Here's how the part is built. I have some questions about the finished solid (model axes, mm). A direction names the side the tool comes from. Coordinates: 2 decimals unless noted, no trailing zeros. Write each loop counter-clockwise with the first axis right and the second up, starting at its lowest first coordinate (ties: lowest second). Pieces come first, ordered by that corner, then holes. Notation, with made-up numbers: M 66,76.25 L 89,76.25 A10 cw 89,85.25 Z; hole C 63.5,-3.5 d5. An arc over 180 degrees is marked long. Write each question's results on one line, items separated by ' | '. Start each with the question number.
from build123d import *

# Parameters (mm, degrees)
F0_W     = 103.023604
F0_H     = 61.1
F0_R     = 2
F1_DEPTH = 2
F2_R     = 5
F3_SIZE  = 0.4


with BuildPart() as f1:
    # F0 (on Top) → F1 (new body)
    with BuildSketch(Plane.XY):
        Rectangle(F0_W, F0_H)
        with Locations((-47.05, -24.27)):
            Circle(F0_R, mode=Mode.SUBTRACT)
        with BuildLine():
            ThreePointArc((49.05, -24.27), (47.05, -26.27), (45.05, -24.27))
            ThreePointArc((45.05, -24.27), (47.05, -22.27), (49.05, -24.27))
        make_face(mode=Mode.SUBTRACT)
        with Locations((-47.05, 24.27)):
            Circle(F0_R, mode=Mode.SUBTRACT)
        Polygon((43.8, -28.2), (-43.8, -28.2), (-43.8, 28.2), (43.8, 28.2), (43.8, -24.27), align=None, mode=Mode.SUBTRACT)
        with Locations((47.05, 24.27)):
            Circle(F0_R, mode=Mode.SUBTRACT)
    extrude(amount=F1_DEPTH)

    # F2
    f2_edges = [f1.edges().sort_by_distance(p)[0] for p in [
        (51.511802, -30.55, 1),
        (51.511802, 30.55, 1),
        (-51.511802, -30.55, 1),
        (-51.511802, 30.55, 1),
    ]]
    fillet(f2_edges, radius=F2_R)

    # F3
    f3_edges = [f1.edges().sort_by_distance(p)[0] for p in [
        (45.05, -24.27, 2),
        (45.05, 24.27, 2),
        (-49.05, 24.27, 2),
        (-49.05, -24.27, 2),
    ]]
    chamfer(f3_edges, length=F3_SIZE)


solid = f1.part
1) I want a section at C-C, the plane y = 8. Write out the boundary of the cut face in (x, z).
2) I want a section at D-D, the plane y = -24.27. Write out the boundary of the cut face in (x, z), then the cut area to 3 significant figures.
3) We'd pull the mould along X, two halves only. Please class faces 1 (the flat face through (-51.512, 0, 1)), 2 (the flat face through (-1, -30.55, 1)), 3 (the cylindrical face through (48.897, 23.504, 0.789)): pulls with the +X half, pulls with the -X half, needs draft (parallel to the pull), parting line crosses it, or undercut.
4) For pin 1 Ø5 at (x, y) = (-47.05, -24.27) entering from -Z, with a flat end and sliding along its axis, tell me the tip position at first contact or that it passes through.
5) I want a section at A-A, the plane x = 2. Write out the boundary of the cut face in (y, z).
6) Please list where these lines run through material, in increasing order: line 1 (Y direction, x = -36, z = 0.15); line 2 (X direction, y = -19.5, z = 0.75); line 3 (Y direction, x = 47.05, z = 0.4). Write a range as [from, to].
7) I want a section at B-B, the plane z = 0.45. Write out the boundary of the cut face in (x, y), then the cut area to 3 significant figures.
8) For faces 4 (the cylindrical face through (50.01, -29.12, 1.01)), 5 (the flat face through (-1, 28.2, 1)), which set-ups out of +Z, -Z, +X, -X, +Y, -Y let a thin tool reach every point of the face, with its end or its side?
Output:
1) outline: M -51.51,0 L -43.8,0 L -43.8,2 L -51.51,2 Z; M 43.8,0 L 51.51,0 L 51.51,2 L 43.8,2 Z
2) outline: M -51.51,0 L -49.05,0 L -49.05,1.6 L -49.45,2 L -51.51,2 Z; M -45.05,0 L -43.8,0 L -43.8,2 L -44.65,2 L -45.05,1.6 Z; M 43.8,0 L 45.05,0 L 45.05,1.6 L 44.65,2 L 43.8,2 Z; M 49.05,0 L 51.51,0 L 51.51,2 L 49.45,2 L 49.05,1.6 Z | area: 14.5 mm2
3) face 1: pulls with the -X half | face 2: needs draft | face 3: undercut
4) pin 1: stops at z = 0
5) outline: M -30.55,0 L -28.2,0 L -28.2,2 L -30.55,2 Z; M 28.2,0 L 30.55,0 L 30.55,2 L 28.2,2 Z
6) line 1: y = [-30.55, -28.2], [28.2, 30.55] | line 2: x = [-51.51, -43.8], [43.8, 51.51] | line 3: y = [-30.52, -26.27], [-22.27, 22.27], [26.27, 30.52]
7) outline: M -51.51,-25.55 A5 ccw -46.51,-30.55 L 46.51,-30.55 A5 ccw 51.51,-25.55 L 51.51,25.55 A5 ccw 46.51,30.55 L -46.51,30.55 A5 ccw -51.51,25.55 Z; hole C -47.05,-24.27 d4; hole C -47.05,24.27 d4; hole M -43.8,-28.2 L 43.8,-28.2 L 43.8,28.2 L -43.8,28.2 Z; hole C 47.05,-24.27 d4; hole C 47.05,24.27 d4 | area: 1,280 mm2
8) face 4: +Z, -Z, +X, -Y | face 5: +Z, -Z
